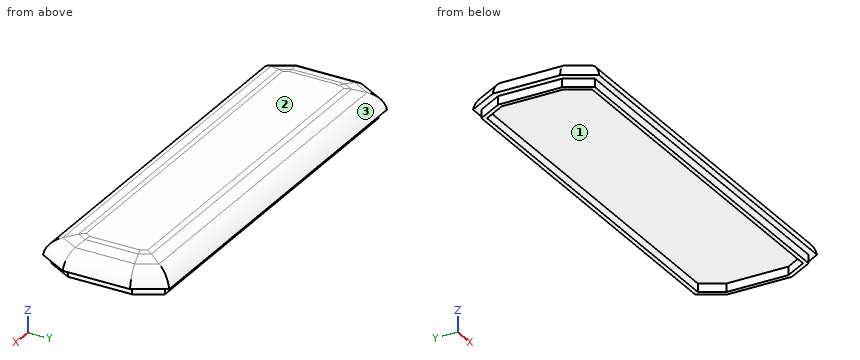
```python
from build123d import *

# Parameters (mm, degrees)
F0_W         = 90
F0_H         = 30
F1_DEPTH     = 5
F2_W         = 1
F2_H         = 2
F4_SIZE2     = 2
F4_SIZE      = 7
F5_T1_DEPTH  = 121.5034235835
F5_T3_DEPTH  = 85.3768581194
F5_T5_DEPTH  = 51.611107996
F5_T7_DEPTH  = 15.783471497
F5_T9_DEPTH  = 71.594276912
F5_T11_DEPTH = 5.6424225565
F5_T13_DEPTH = 51.611107996
F5_T15_DEPTH = 5.6424225565
F5_T17_DEPTH = 51.611107996
F5_T19_DEPTH = 5.6424225565
F5_T21_DEPTH = 5.6424225565
F5_T23_DEPTH = 51.611107996


# Not quite as in the source:
# - a fillet or chamfer that OpenCascade refuses, or shapes differently, is made with other operations: its cross-section is extruded or revolved along the edge and cut away or added


with BuildPart() as f1:
    # F0 (on Top) → F1 (new body)
    with BuildSketch(Plane.XY):
        Polygon((-45, -15), (-45, 15), (-49, 8), (-49, -8), align=None)
        Polygon((49, 8), (45, 15), (45, -15), (49, -8), align=None)
        Rectangle(F0_W, F0_H)
    extrude(amount=F1_DEPTH)

    # F3: sweep along a path in F3_path
    with BuildLine(Plane(origin=(45, -15, 0), x_dir=(0, -1, 0), z_dir=(0, 0, -1))) as f3_path:
        Line((0, 0), (0, 90))
        Line((0, 90), (-7, 94))
        Line((-7, 94), (-23, 94))
        Line((-23, 94), (-30, 90))
        Line((-30, 90), (-30, 0))
        Line((-30, 0), (-23, -4))
        Line((-23, -4), (-7, -4))
        Line((-7, -4), (0, 0))
    # F2 (on Right) → F3 (sweep)
    with BuildSketch(Plane.YZ):
        with Locations((-13, -1)):
            Rectangle(F2_W, F2_H)
    sweep(path=f3_path.line, transition=Transition.RIGHT)

    # F4
    f4_edges = [f1.edges().sort_by_distance(p)[0] for p in [
        (-49, 0, 5),
        (-47, -11.5, 5),
        (-47, 11.5, 5),
        (47, -11.5, 5),
        (49, 0, 5),
        (47, 11.5, 5),
        (0, -15, 5),
        (0, 15, 5),
    ]]
    f4_side = f1.faces().sort_by_distance((0, 0, 5))[0]
    chamfer(f4_edges, length=F4_SIZE, length2=F4_SIZE2, reference=f4_side)

    # F5: fillet of radius 5 on 16 edges, made by hand

    # F5_s2 → F5_t1 (cut)
    with BuildSketch(Plane.YZ.offset(-60.7517117917)):
        with BuildLine():
            ThreePointArc((15, 0), (13.8034764966, 2.5282074371), (11.4363180932, 4.0181948305))
            Line((11.4363180932, 4.0181948305), (15, 3))
            Line((15, 3), (15, 0))
        make_face()
        with BuildLine():
            ThreePointArc((-15, 0), (-13.8034764966, 2.5282074371), (-11.4363180932, 4.0181948305))
            Line((-11.4363180932, 4.0181948305), (-15, 3))
            Line((-15, 3), (-15, 0))
        make_face()
    extrude(amount=F5_T1_DEPTH, mode=Mode.SUBTRACT)

    # F5_s4 → F5_t3 (cut)
    with BuildSketch(Plane.YZ.offset(-42.6884290597)):
        with BuildLine():
            ThreePointArc((8.6733309163, 4.8076197382), (7.9932313362, 4.9516713689), (7.2997252768, 5))
            Line((7.2997252768, 5), (8, 5))
            Line((8, 5), (8.6733309163, 4.8076197382))
        make_face()
        with BuildLine():
            ThreePointArc((-7.2997252768, 5), (-7.9932313362, 4.9516713689), (-8.6733309163, 4.8076197382))
            Line((-8.6733309163, 4.8076197382), (-8, 5))
            Line((-8, 5), (-7.2997252768, 5))
        make_face()
    extrude(amount=F5_T3_DEPTH, mode=Mode.SUBTRACT)

    # F5_s6 → F5_t5 (cut)
    with BuildSketch(Plane(origin=(-22.4066273783, 39.211597912, 0), x_dir=(0, 0, 1), z_dir=(0.4961389384, -0.8682431421, 0))):
        with BuildLine():
            ThreePointArc((0, 46.513025471), (2.5282074371, 45.3165019675), (4.0181948305, 42.9493435641))
            Line((4.0181948305, 42.9493435641), (3, 46.513025471))
            Line((3, 46.513025471), (0, 46.513025471))
        make_face()
    extrude(amount=F5_T5_DEPTH, mode=Mode.SUBTRACT)

    # F5_s8 → F5_t7 (cut)
    with BuildSketch(Plane.XZ.offset(-7.8917357485)):
        with BuildLine():
            ThreePointArc((-41.2997252768, 5), (-41.9932313362, 4.9516713689), (-42.6733309163, 4.8076197382))
            Line((-42.6733309163, 4.8076197382), (-42, 5))
            Line((-42, 5), (-41.2997252768, 5))
        make_face()
        with BuildLine():
            ThreePointArc((41.2997252768, 5), (41.9932313362, 4.9516713689), (42.6733309163, 4.8076197382))
            Line((42.6733309163, 4.8076197382), (42, 5))
            Line((42, 5), (41.2997252768, 5))
        make_face()
    extrude(amount=F5_T7_DEPTH, mode=Mode.SUBTRACT)

    # F5_s10 → F5_t9 (cut)
    with BuildSketch(Plane.XZ.offset(-35.797138456)):
        with BuildLine():
            ThreePointArc((-49, 0), (-47.8034764966, 2.5282074371), (-45.4363180932, 4.0181948305))
            Line((-45.4363180932, 4.0181948305), (-49, 3))
            Line((-49, 3), (-49, 0))
        make_face()
        with BuildLine():
            ThreePointArc((49, 0), (47.8034764966, 2.5282074371), (45.4363180932, 4.0181948305))
            Line((45.4363180932, 4.0181948305), (49, 3))
            Line((49, 3), (49, 0))
        make_face()
    extrude(amount=F5_T9_DEPTH, mode=Mode.SUBTRACT)

    # F5_s12 → F5_t11 (cut)
    with BuildSketch(Plane(origin=(-8.5616705046, 14.982923383, 0), x_dir=(0, 0, 1), z_dir=(0.4961389384, -0.8682431421, 0))):
        with BuildLine():
            ThreePointArc((5, 38.8127507478), (4.9516713689, 39.5062568072), (4.8076197382, 40.1863563872))
            Line((4.8076197382, 40.1863563872), (5, 39.513025471))
            Line((5, 39.513025471), (5, 38.8127507478))
        make_face()
    extrude(amount=F5_T11_DEPTH, mode=Mode.SUBTRACT)

    # F5_s14 → F5_t13 (cut)
    with BuildSketch(Plane(origin=(3.1996529503, 5.599392663, 0), x_dir=(0, 0, 1), z_dir=(-0.4961389384, -0.8682431421, 0))):
        with BuildLine():
            ThreePointArc((0, 46.513025471), (2.5282074371, 45.3165019675), (4.0181948305, 42.9493435641))
            Line((4.0181948305, 42.9493435641), (3, 46.513025471))
            Line((3, 46.513025471), (0, 46.513025471))
        make_face()
    extrude(amount=F5_T13_DEPTH, mode=Mode.SUBTRACT)

    # F5_s16 → F5_t15 (cut)
    with BuildSketch(Plane(origin=(-5.7622449676, -10.0839286934, 0), x_dir=(0, 0, 1), z_dir=(-0.4961389384, -0.8682431421, 0))):
        with BuildLine():
            ThreePointArc((4.8076197382, 40.1863563872), (4.9516713689, 39.5062568072), (5, 38.8127507478))
            Line((5, 38.8127507478), (5, 39.513025471))
            Line((5, 39.513025471), (4.8076197382, 40.1863563872))
        make_face()
    extrude(amount=F5_T15_DEPTH, mode=Mode.SUBTRACT)

    # F5_s18 → F5_t17 (cut)
    with BuildSketch(Plane(origin=(22.4066273783, -39.211597912, 0), x_dir=(0, 0, 1), z_dir=(-0.4961389384, 0.8682431421, 0))):
        with BuildLine():
            ThreePointArc((0, 46.513025471), (2.5282074371, 45.3165019675), (4.0181948305, 42.9493435641))
            Line((4.0181948305, 42.9493435641), (3, 46.513025471))
            Line((3, 46.513025471), (0, 46.513025471))
        make_face()
    extrude(amount=F5_T17_DEPTH, mode=Mode.SUBTRACT)

    # F5_s20 → F5_t19 (cut)
    with BuildSketch(Plane(origin=(8.5616705046, -14.982923383, 0), x_dir=(0, 0, 1), z_dir=(-0.4961389384, 0.8682431421, 0))):
        with BuildLine():
            ThreePointArc((5, 38.8127507478), (4.9516713689, 39.5062568072), (4.8076197382, 40.1863563872))
            Line((4.8076197382, 40.1863563872), (5, 39.513025471))
            Line((5, 39.513025471), (5, 38.8127507478))
        make_face()
    extrude(amount=F5_T19_DEPTH, mode=Mode.SUBTRACT)

    # F5_s22 → F5_t21 (cut)
    with BuildSketch(Plane(origin=(5.7622449676, 10.0839286934, 0), x_dir=(0, 0, 1), z_dir=(0.4961389384, 0.8682431421, 0))):
        with BuildLine():
            ThreePointArc((5, 38.8127507478), (4.9516713689, 39.5062568072), (4.8076197382, 40.1863563872))
            Line((4.8076197382, 40.1863563872), (5, 39.513025471))
            Line((5, 39.513025471), (5, 38.8127507478))
        make_face()
    extrude(amount=F5_T21_DEPTH, mode=Mode.SUBTRACT)

    # F5_s24 → F5_t23 (cut)
    with BuildSketch(Plane(origin=(-3.1996529503, -5.599392663, 0), x_dir=(0, 0, 1), z_dir=(0.4961389384, 0.8682431421, 0))):
        with BuildLine():
            ThreePointArc((0, 46.513025471), (2.5282074371, 45.3165019675), (4.0181948305, 42.9493435641))
            Line((4.0181948305, 42.9493435641), (3, 46.513025471))
            Line((3, 46.513025471), (0, 46.513025471))
        make_face()
    extrude(amount=F5_T23_DEPTH, mode=Mode.SUBTRACT)


solid = f1.part
```
Input: part model. Units: mm. Frame: model coordinates. Face numbers are marked on the shaded views. Coordinates: 2 decimals unless noted, no trailing zeros. Order: outer loops, then holes, each group sorted by start corner. A loop starts at its lowest first (then second) coordinate and runs counter-clockwise, first axis right, second up. Notation, with made-up numbers: (62, 26.5) - (107, 26.5) arc R27 ccw to (107, 47.5) - close; hole circle Ø6 at (81.5, 0.5). An arc over 180 degrees is marked (long way). Put each result on its own line as item: value.
1. Line query: line 1 along Y through (x, z) = (10.5, -1.5); line 2 along X through (y, z) = (3, -1.5); line 3 along Z through (x, y) = (13.5, 1.5). Output: solid intervals per line, ascending.
Report:
line 1: y = -13.5 to -12.5, 12.5 to 13.5
line 2: x = -47.5 to -46.5, 46.5 to 47.5
line 3: z = 0 to 5
2. Contact query for flat-ended pins moving along their axis: pin 1 Ø1.5 at (y, z) = (-2, -1) entering from -X; pin 2 Ø5 at (x, y) = (-23.5, -8.5) entering from -Z; pin 3 Ø1 at (x, z) = (18.5, -1) entering from -Y. Output: stop coordinate, or through.
Report:
pin 1: stops at x = -47.5
pin 2: stops at z = 0
pin 3: stops at y = -13.5
3. Cut plane A-A on z = -1. Return the cut outline in (x, y), then the cut area to 3 significant figures.
Report:
outline: (-47.5, -7.6) - (-44.13, -13.5) - (44.13, -13.5) - (47.5, -7.6) - (47.5, 7.6) - (44.13, 13.5) - (-44.13, 13.5) - (-47.5, 7.6) - close; hole (-46.5, -7.34) - (-43.55, -12.5) - (43.55, -12.5) - (46.5, -7.34) - (46.5, 7.34) - (43.55, 12.5) - (-43.55, 12.5) - (-46.5, 7.34) - close
area: 231 mm2
4. Cut plane B-B on y = 4. Return the cut outline in (x, z), then the cut area to 3 significant figures.
Report:
outline: (-49, 0) - (-47.5, 0) - (-47.5, -2) - (-46.5, -2) - (-46.5, 0) - (46.5, 0) - (46.5, -2) - (47.5, -2) - (47.5, 0) - (49, 0) arc R5 ccw to (45.44, 4.02) - (42.67, 4.81) arc R5 ccw to (41.3, 5) - (-41.3, 5) arc R5 ccw to (-42.67, 4.81) - (-45.44, 4.02) arc R5 ccw to start
area: 475 mm2
5. Draft query along Y for the marked faces 1, 2 and 3. Return one class per face: pulls with the +Y half, pulls with the -Y half, needs draft (parallel to the pull), parting line crosses it, or undercut.
Report:
face 1: undercut
face 2: needs draft
face 3: pulls with the +Y half
6. Cut plane D-D on z = 3. Return the cut outline in (x, y), then the cut area to 3 significant figures.
Report:
outline: (-47.32, -7.56) - (-44.03, -13.32) - (44.03, -13.32) - (47.32, -7.56) - (47.32, 7.56) - (44.03, 13.32) - (-44.03, 13.32) - (-47.32, 7.56) - close
area: 2,480 mm2
7. Cut plane C-C on x = -32. Return the cut outline in (y, z), then the cut area to 3 significant figures.
Report:
outline: (-15, 0) - (-13.5, 0) - (-13.5, -2) - (-12.5, -2) - (-12.5, 0) - (12.5, 0) - (12.5, -2) - (13.5, -2) - (13.5, 0) - (15, 0) arc R5 ccw to (11.44, 4.02) - (8.67, 4.81) arc R5 ccw to (7.3, 5) - (-7.3, 5) arc R5 ccw to (-8.67, 4.81) - (-11.44, 4.02) arc R5 ccw to start
area: 135 mm2
